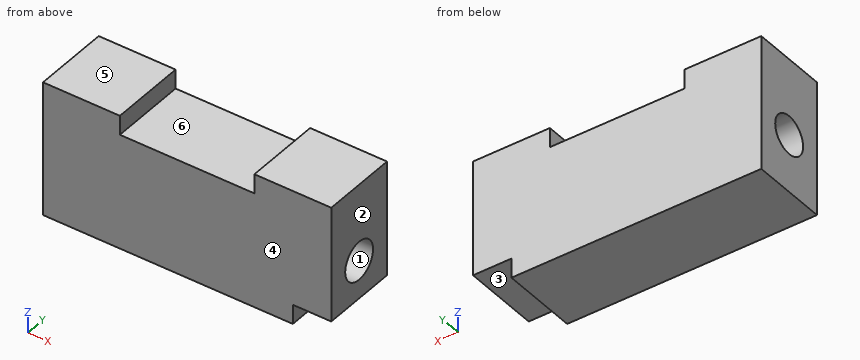
```python
from build123d import *

# Parameters (mm, degrees)
F0_W     = 82.55
F0_H     = 38.1
F2_DEPTH = 12.7
F3_W     = 25.4
F3_H     = 25.4
F4_DEPTH = 6.35
F5_W     = 25.4
F5_H     = 6.416842
F5_H_2   = 31.683158
F6_DEPTH = 12.7
F7_R     = 6.35
F8_DEPTH = 95.251


with BuildPart() as f2:
    # F0 (on Front) → F2 (new body, symmetric)
    with BuildSketch(Plane.XZ):
        Rectangle(F0_W, F0_H)
    extrude(amount=F2_DEPTH, both=True)

    # F3 (on face) → F4 (join, symmetric)
    with BuildSketch(Plane.XY.offset(19.05)):
        with Locations((-28.575, 0)):
            Rectangle(F3_W, F3_H)
    extrude(amount=F4_DEPTH, both=True)

    # F5 (on face) → F6 (join, symmetric)
    with BuildSketch(Plane.YZ.offset(41.275)):
        with Locations((0, 22.258421)):
            Rectangle(F5_W, F5_H)
        with Locations((0, 3.208421)):
            Rectangle(F5_W, F5_H_2)
    extrude(amount=F6_DEPTH, both=True)

    # F7 (on face) → F8 (cut, through all)
    with BuildSketch(Plane.YZ.offset(53.975)):
        Circle(F7_R)
    extrude(amount=-F8_DEPTH, mode=Mode.SUBTRACT)


solid = f2.part
```
For this review, take the finished solid that the model builds, in its own axes (mm). Face numbers are marked on the shaded views. A direction names the side the tool comes from. Coordinates: 2 decimals unless noted, no trailing zeros. Order: outer loops, then holes, each group sorted by start corner. A loop starts at its lowest first (then second) coordinate and runs counter-clockwise, first axis right, second up. Notation, with made-up numbers: (-29, 8.5) -> (-15, 8.5) arc R25 cw to (-15, 36.5) -> close; hole circle Ø6 at (13.25, -3.5). An arc over 180 degrees is marked (long way). Use CSV: the item, a comma, the result in double quotes. Start each with the question number.
Item 1: Wall thickness on probe 1 along X at (y, z) = (-7.75, 24.5) (3 decimals); probe 2 along Z at (x, y) = (11, 0); probe 3 along X at (y, z) = (-6.5, -17) (3 decimals): over which ranges is each line inside the solid? List them lowest first.
Item 2: We need section B-B, the plane x = -25.5. Give the boundary of the cut face in (y, z), then the cut area to 3 significant figures.
Item 3: We need section C-C, the plane y = 0. Give the boundary of the cut face in (x, z) (3 decimals).
Item 4: For the marked faces 4, 5 and 6, list the 3-axis set-ups (+Z, -Z, +X, -X, +Y, -Y) from which the entire face can be reached by the end or side of a thin tool; tool diameter is ignored.
Item 5: We need section D-D, the plane y = -8. Give the boundary of the cut face in (x, z) (3 decimals).
Item 6: We need section A-A, the plane z = 21.5. Give the boundary of the cut face in (x, y) (3 decimals).
Item 7: Draft analysis for pull direction Z (two halves, no side actions). For the marked faces 1, 2 and 3, state which applies: pulls with the +Z half, pulls with the -Z half, needs draft (parallel to the pull), parting line crosses it, or undercut.
Item 8: Insertion check: pin 1 (7.5 mm diameter, centred on x = -4, y = 3.5, fed in from +Z); pin 2 (4 mm diameter, centred on x = 46.5, y = -3, fed in from -Z); pin 3 (4 mm diameter, centred on x = 12.5, y = 6, fed in from +Z). Each pin has a flat end and moves straight along its axis. Give the tip position at first contact, or say it passes through.
Derived:
1,probe 1,"x = -41.275 to -15.875, 28.575 to 53.975"
1,probe 2,"z = -19.05 to -6.35, 6.35 to 19.05"
1,probe 3,"x = -41.275 to 41.275"
2,outline,"(-12.7, -19.05) -> (12.7, -19.05) -> (12.7, 25.4) -> (-12.7, 25.4) -> close; hole circle Ø12.7 at (0, 0)"
2,area,"1,000 mm^2"
3,outline,"(-41.275, -19.05) -> (41.275, -19.05) -> (41.275, -12.633) -> (53.975, -12.633) -> (53.975, -6.35) -> (-41.275, -6.35) -> close; (-41.275, 6.35) -> (53.975, 6.35) -> (53.975, 25.467) -> (28.575, 25.467) -> (28.575, 19.05) -> (-15.875, 19.05) -> (-15.875, 25.4) -> (-41.275, 25.4) -> close"
4,face 4,"+Z, -Z, +X, -X, -Y"
4,face 5,"+Z, -X, +Y, -Y"
4,face 6,"+Z, +Y, -Y"
5,outline,"(-41.275, -19.05) -> (41.275, -19.05) -> (41.275, -12.633) -> (53.975, -12.633) -> (53.975, 25.467) -> (28.575, 25.467) -> (28.575, 19.05) -> (-15.875, 19.05) -> (-15.875, 25.4) -> (-41.275, 25.4) -> close"
6,outline,"(-41.275, -12.7) -> (-15.875, -12.7) -> (-15.875, 12.7) -> (-41.275, 12.7) -> close; (28.575, -12.7) -> (53.975, -12.7) -> (53.975, 12.7) -> (28.575, 12.7) -> close"
7,face 1,"undercut"
7,face 2,"needs draft"
7,face 3,"pulls with the -Z half"
8,pin 1,"stops at z = 19.05"
8,pin 2,"stops at z = -12.63"
8,pin 3,"stops at z = 19.05"
